Work out the finished part from the listing and answer in its coordinate system (mm). Face numbers are marked on the shaded views. A direction names the side the tool comes from. Round coordinates to 2 decimals unless told otherwise and drop trailing zeros. Write each loop counter-clockwise with the first axis right and the second up, starting at its lowest first coordinate (ties: lowest second). Pieces come first, ordered by that corner, then holes. Notation, with made-up numbers: M 56.25,24 L 93.25,24 A18 ccw 93.25,34 Z; hole C 22.25,-38 d4. An arc over 180 degrees is marked long. One line per item, written item: value. Start each with the question number.
Q1. A tool of negligible diameter and unlimited length cuts with its end or side. For the marked faces 1 and 2, from which of +Z, -Z, +X, -X, +Y, -Y can it reach the whole face along a straight path? Write none if from no direction.
Q2. Find section A-A (z = -1.25). Write down the section's boundary in (x, y).
Q3. Consider probe 1 along X at (y, z) = (-33, -2.5); probe 2 along Z at (x, y) = (0, 3); probe 3 along Z at (x, y) = (-62.5, -33.5). Determine where each line is inside the solid, lowest interval first.
Q4. Find section B-B (y = -9). Write down the section's boundary in (x, z).
Q5. Find section D-D (x = -49). Write down the section's boundary in (y, z), and give its area (3 significant figures).
Q6. Find section C-C (x = -13). Write down the section's boundary in (y, z).
Q7. Given pin 1 Ø5 at (x, z) = (-2.5, -2.5) entering from -Y; pin 2 Ø4 at (y, z) = (-26, -1) entering from +X; pin 3 Ø22 at (x, y) = (-44.5, 4) entering from -Z; pin 4 Ø3 at (x, z) = (-57, 4.5) entering from -Y, each flat-ended and moving along its own axis, determine where each tip first touches the part or whether it passes through.
from build123d import *

# Parameters (mm, degrees)
SALIENTE_EXTRUIR1_DEPTH = 10
CROQUIS2_R              = 2.6
CORTAR_EXTRUIR1_DEPTH   = 21
CROQUIS3_R              = 4
SALIENTE_EXTRUIR2_DEPTH = 30
CROQUIS4_R              = 2.6
CORTAR_EXTRUIR2_DEPTH   = 10
SALIENTE_EXTRUIR3_START = -13
CROQUIS5_R              = 6.5
SALIENTE_EXTRUIR3_DEPTH = 3


with BuildPart() as part:
    # Croquis1 → Saliente-Extruir1 (new body, symmetric)
    with BuildSketch(Plane(origin=(0, 0, 0), x_dir=(1, 0, 0), z_dir=(0, 1, 0))):
        with BuildLine():
            Line((-62.5, 6.5), (0, 6.5))
            ThreePointArc((0, 6.5), (6.494806232, -0.259792249), (-0.519169329, -6.479233227))
            Line((-0.519169329, -6.479233227), (-62.819488818, -1.487220447))
            ThreePointArc((-62.819488818, -1.487220447), (-66.496803835, 2.659872153), (-62.5, 6.5))
        make_face()
    extrude(amount=SALIENTE_EXTRUIR1_DEPTH, both=True)

    # Croquis2 → Cortar-Extruir1 (cut, through all)
    with BuildSketch(Plane(origin=(0, 10, 0), x_dir=(1, 0, 0), z_dir=(0, 1, 0))):
        Circle(CROQUIS2_R)
    extrude(amount=-CORTAR_EXTRUIR1_DEPTH, mode=Mode.SUBTRACT)

    # Croquis3 → Saliente-Extruir2 (add)
    with BuildSketch(Plane(origin=(0, -10, 0), x_dir=(1, 0, 0), z_dir=(0, 1, 0))):
        with Locations((-62.5, 2.5)):
            Circle(CROQUIS3_R)
    extrude(amount=-SALIENTE_EXTRUIR2_DEPTH)

    # Croquis4 → Cortar-Extruir2 (cut)
    with BuildSketch(Plane(origin=(0, -40, 0), x_dir=(-1, 0, 0), z_dir=(0, -1, 0))):
        with Locations((62.5, 2.5)):
            Circle(CROQUIS4_R)
    extrude(amount=-CORTAR_EXTRUIR2_DEPTH, mode=Mode.SUBTRACT)

    # Croquis5 → Saliente-Extruir3 (add)
    with BuildSketch(Plane.XZ.offset(40).offset(SALIENTE_EXTRUIR3_START)):
        with Locations((-62.5, -2.5)):
            Circle(CROQUIS5_R)
    extrude(amount=SALIENTE_EXTRUIR3_DEPTH)


solid = part.part
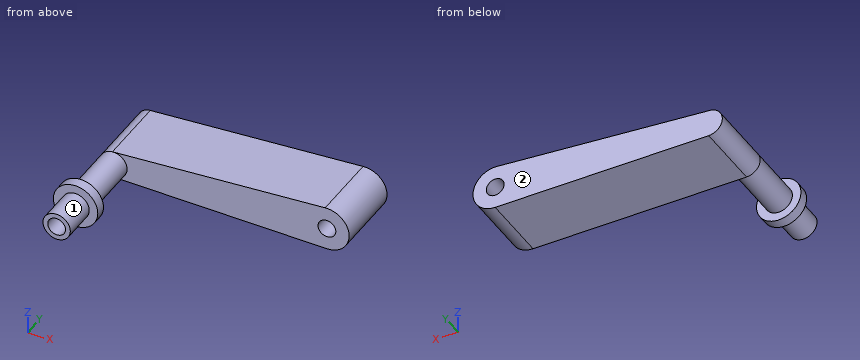
The answers:
1. face 1: -Y
1. face 2: +Z, -Z, +X, -X, +Y
2. outline: M -68.88,-30 L -66.3,-30 L -66.3,-40 L -64.78,-40 L -64.78,-30 L -60.22,-30 L -60.22,-40 L -58.7,-40 L -58.7,-30 L -56.12,-30 L -56.12,-27 L -58.7,-27 L -58.7,-10 L -2.28,-10 L -2.28,10 L -66.3,10 L -66.3,-27 L -68.88,-27 Z; M 2.28,-10 L 6.38,-10 L 6.38,10 L 2.28,10 Z
3. probe 1: -66.5 to -65.1, -59.9 to -58.5
3. probe 2: -6.5 to -2.6, 2.6 to 6.5
3. probe 3: -6.5 to -5.1, 0.1 to 1.5
4. outline: M -62.82,1.49 A4 ccw -62.5,-6.5 L 0,-6.5 A6.5 ccw long -0.52,6.48 Z; hole C 0,0 d5.2
5. outline: M -10,-6.5 L 10,-6.5 L 10,2.59 L -10,2.59 Z
5. area: 182 mm2
6. outline: M -10,-6.5 L 10,-6.5 L 10,5.48 L -10,5.48 Z
7. pin 1: y = -10
7. pin 2: x = -56
7. pin 3: z = -6.5
7. pin 4: through
